Could you check a few things on this drawing? It's one solid part, dimensions in mm from its lowest x, y, z. Give positions to 0.01 mm unless a question says otherwise; leave off trailing zeros. Loops run counter-clockwise (first coordinate to the right, second up) from the corner with the lowest first, then second, coordinate; pieces in that order, holes last.
1. I need wall thicknesses on line 1 along X through (y, z) = (0.75, 64); line 2 along Z through (x, y) = (136, 4.3); line 3 along Z through (x, y) = (145.5, 1.6). Which ranges of each line are inside material? Lowest first, please.
2. Imagine slicing it at C-C (y = 2.55). List the corners of the cut face in (x, z) for me, plus the area to 3 significant figures.
3. Imagine slicing it at B-B (x = 79.5). List the corners of the cut face in (y, z) for me.
4. Imagine slicing it at A-A (z = 117.5). List the corners of the cut face in (x, y) for me, plus the area to 3 significant figures.
5. Imagine slicing it at D-D (x = 144). List the corners of the cut face in (y, z) for me, plus the area to 3 significant figures.
6. For P1, Ø3, axis at x = 118.5, y = 2.5, coming from the -Z side; P2, Ø8, axis at x = 53.5, z = 154.5, coming from the +Y side, each with a flat end and sliding along its axis, tell me the tip position at first contact or that it passes through.
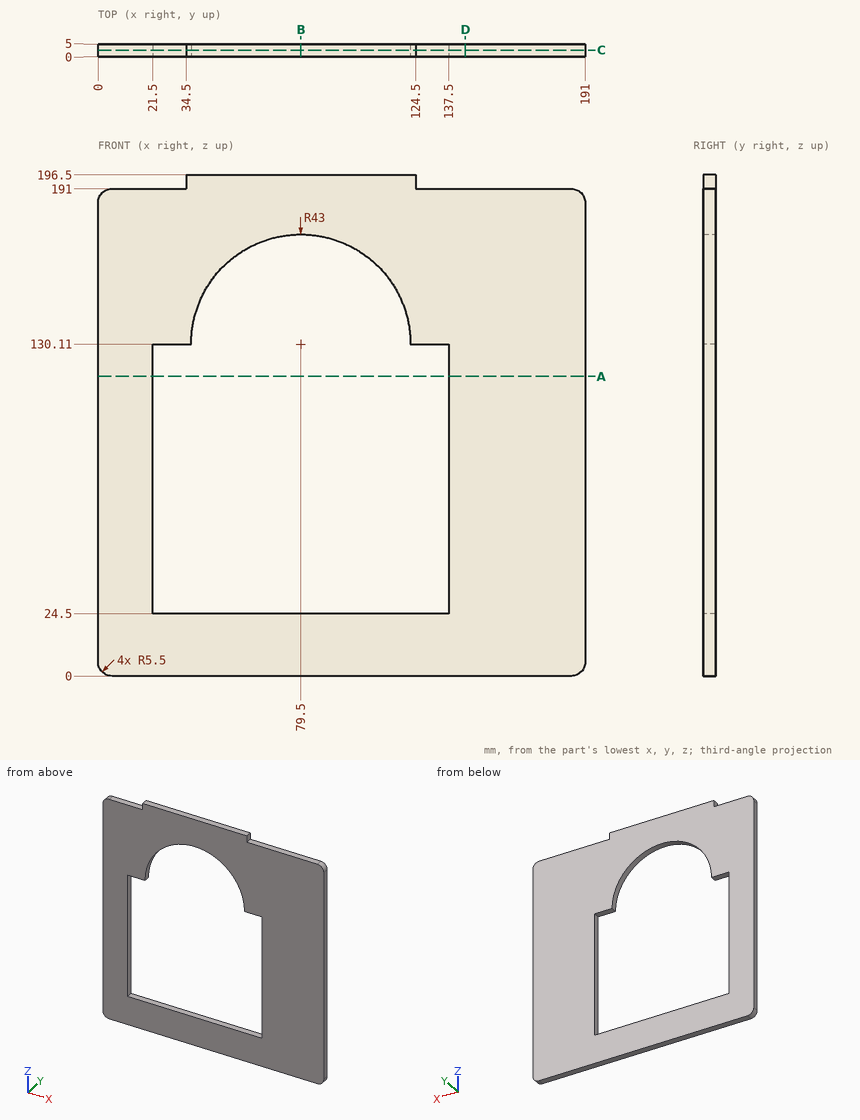
Derived:
1. line 1: x = 0 to 21.5, 137.5 to 191
1. line 2: z = 0 to 24.5, 130.11 to 191
1. line 3: z = 0 to 191
2. outline: (0, 5.5) arc R5.5 ccw to (5.5, 0) - (185.5, 0) arc R5.5 ccw to (191, 5.5) - (191, 185.5) arc R5.5 ccw to (185.5, 191) - (124.5, 191) - (124.5, 196.5) - (34.5, 196.5) - (34.5, 191) - (5.5, 191) arc R5.5 ccw to (0, 185.5) - close; hole (21.5, 24.5) - (137.5, 24.5) - (137.5, 130.11) - (122.5, 130.11) arc R43 ccw to (36.5, 130.11) - (21.5, 130.11) - close
2. area: 21,800 mm2
3. outline: (0, 0) - (5, 0) - (5, 24.5) - (0, 24.5) - close; (0, 173.11) - (5, 173.11) - (5, 196.5) - (0, 196.5) - close
4. outline: (0, 0) - (21.5, 0) - (21.5, 5) - (0, 5) - close; (137.5, 0) - (191, 0) - (191, 5) - (137.5, 5) - close
4. area: 375 mm2
5. outline: (0, 0) - (5, 0) - (5, 191) - (0, 191) - close
5. area: 955 mm2
6. P1: stops at z = 0
6. P2: passes through
